Input: part model. Units: mm. Frame: model coordinates. Face numbers are marked on the shaded views. A direction names the side the tool comes from. Give positions to 0.01 mm unless a question says otherwise; leave off trailing zeros. Write each loop counter-clockwise with the first axis right and the second up, starting at its lowest first coordinate (ties: lowest second). Pieces come first, ordered by that corner, then holes. Notation, with made-up numbers: (77.5, -34.5) -> (97.5, -34.5) arc R13 ccw to (97.5, -19.5) -> close; hole circle Ø4 at (2, 25.5). An arc over 180 degrees is marked (long way). Answer as a JSON object with one key per item and string values. Group by question number.
from build123d import *

# Parameters (mm, degrees)
BOSS_EXTRUDE1_DEPTH = 5
SKETCH2_R           = 1.5
CUT_EXTRUDE1_DEPTH  = 5
SKETCH1_4_OUTSIDE_W = 53.856
SKETCH1_4_OUTSIDE_H = 58.288
SKETCH1_4_OUTSIDE_R = 1.5
CUT_EXTRUDE3_DEPTH  = 31.230173018
BOSS_EXTRUDE2_DEPTH = 40
SKETCH5_W           = 5
SKETCH5_H           = 50
BOSS_EXTRUDE3_DEPTH = 40
BOSS_EXTRUDE4_DEPTH = 40
SKETCH9_R           = 2
CUT_EXTRUDE4_DEPTH  = 84.384553352


with BuildPart() as part:
    # Sketch1 → Boss-Extrude1 (new body)
    with BuildSketch(Plane(origin=(0, 0, 0), x_dir=(1, 0, 0), z_dir=(0, 1, 0))):
        Polygon((-14.94438846, 22.160431622), (14.94438846, 22.160431622), (19.94438846, 17.160431622), (19.94438846, -22.160431622), (-19.94438846, -22.160431622), (-19.94438846, 17.160431622), align=None)
    extrude(amount=BOSS_EXTRUDE1_DEPTH)

    # Sketch2 → Cut-Extrude1 (cut)
    with BuildSketch(Plane.XZ):
        with Locations(Location((-8.780710157, 0, 0), (0, 0, 270))):
            Circle(SKETCH2_R)
    extrude(amount=-CUT_EXTRUDE1_DEPTH, mode=Mode.SUBTRACT)

    # Sketch1_4 outside → Cut-Extrude3 (cut, through all)
    # profile 1 of 3: a face of its own
    with BuildSketch(Plane(origin=(0, 0, 0), x_dir=(1, 0, 0), z_dir=(0, 1, 0))):
        Rectangle(SKETCH1_4_OUTSIDE_W, SKETCH1_4_OUTSIDE_H)
        Polygon((-14.94438846, 22.160431622), (14.94438846, 22.160431622), (19.94438846, 17.160431622), (19.94438846, -22.160431622), (-19.94438846, -22.160431622), (-19.94438846, 17.160431622), align=None, mode=Mode.SUBTRACT)
    # profile 2 of 3: a face of its own
    with BuildSketch(Plane(origin=(0, 0, 0), x_dir=(1, 0, 0), z_dir=(0, 1, 0))):
        with Locations(Location((8.788189679, 0, 0), (0, 0, 270))):
            Circle(SKETCH1_4_OUTSIDE_R)
    # profile 3 of 3: a face of its own
    with BuildSketch(Plane(origin=(0, 0, 0), x_dir=(1, 0, 0), z_dir=(0, 1, 0))):
        with Locations((-8.788189679, 0)):
            Circle(SKETCH1_4_OUTSIDE_R)
    extrude(amount=CUT_EXTRUDE3_DEPTH, mode=Mode.SUBTRACT)

    # Sketch4 → Boss-Extrude2 (add)
    with BuildSketch(Plane(origin=(19.94438846, 0, 0), x_dir=(0, 0, -1), z_dir=(1, 0, 0))):
        with BuildLine():
            Line((-22.160431622, 5), (-22.160431622, 0))
            ThreePointArc((-22.160431622, 0), (-29.231499434, 2.928932188), (-32.160431622, 10))
            Line((-32.160431622, 10), (-27.160431622, 10))
            ThreePointArc((-27.160431622, 10), (-25.695965528, 6.464466094), (-22.160431622, 5))
        make_face()
    extrude(amount=-BOSS_EXTRUDE2_DEPTH)

    # Sketch5 → Boss-Extrude3 (add)
    with BuildSketch(Plane(origin=(19.94438846, 0, 0), x_dir=(0, 0, -1), z_dir=(1, 0, 0))):
        with Locations((-29.660431622, 35)):
            Rectangle(SKETCH5_W, SKETCH5_H)
    extrude(amount=-BOSS_EXTRUDE3_DEPTH)

    # Sketch6 → Boss-Extrude4 (add)
    with BuildSketch(Plane(origin=(19.94438846, 0, 0), x_dir=(0, 0, -1), z_dir=(1, 0, 0))):
        Polygon((-10.08936381, 5), (-18.624897716, 13.535533906), (-27.160431622, 22.071067812), (-27.160431622, 17.071067812), (-15.08936381, 5), align=None)
    extrude(amount=-BOSS_EXTRUDE4_DEPTH)

    # Sketch9 → Cut-Extrude4 (cut, through all)
    with BuildSketch(Plane.XY.offset(32.160431622)):
        with Locations((-0.05561154, 46)):
            Circle(SKETCH9_R)
    extrude(amount=-CUT_EXTRUDE4_DEPTH, mode=Mode.SUBTRACT)


solid = part.part
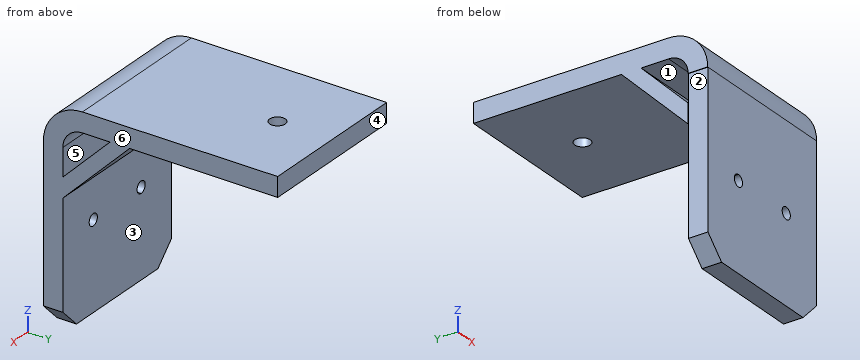
1. Reachability of the marked faces 1, 2 and 3 from +Z, -Z, +X, -X, +Y, -Y: full face, straight path, thin tool, end or side. Return the list, or none.
2. Contact query for flat-ended pins moving along their axis: pin 1 Ø1.5 at (y, z) = (2.5, -6.5) entering from -X; pin 2 Ø11.5 at (x, y) = (6.5, 44.5) entering from -Z; pin 3 Ø10 at (x, y) = (9, 23.5) entering from -Z; pin 4 Ø1.8 at (x, z) = (8.79, 0) entering from -Y. Output: stop coordinate, or through.
3. Section B-B (z = 0). Return the cut outline in (x, y).
4. Mould query, pull axis Y, two halves, no side actions, for the marked faces 4, 5 and 6. Classes: pulls with the +Y half, pulls with the -Y half, needs draft (parallel to the pull), parting line crosses it, or undercut.
5. Section C-C (y = 46). Return the cut outline in (x, z), plus the area to 3 significant figures.
6. Line query: line 1 (X direction, y = 1, z = 0); line 2 (Z direction, x = -14, y = 52); line 3 (Y direction, x = -17, z = -7). Output: solid intervals per line, ascending.
7. Section D-D (x = 0). Return the cut outline in (y, z), plus the area to 3 significant figures.
8. Section A-A (x = 14). Return the cut outline in (y, z).
Working result:
{
 "1": {"face 1": "+X, -X", "face 2": "-Z, -X, -Y", "face 3": "-Z, +X, -X, +Y"},
 "2": {"pin 1": "stops at x = -19.94", "pin 2": "stops at z = 27.16", "pin 3": "stops at z = 23.59", "pin 4": "passes through"},
 "3": {"outline": "(-19.94, 0) -> (-10.29, 0) -> (-10.29, 5) -> (-19.94, 5) -> close; (-7.28, 0) -> (7.29, 0) -> (7.29, 5) -> (-7.28, 5) -> close; (10.29, 0) -> (19.94, 0) -> (19.94, 5) -> (10.29, 5) -> close"},
 "4": {"face 4": "pulls with the +Y half", "face 5": "undercut", "face 6": "needs draft"},
 "5": {"outline": "(-20.06, 27.16) -> (-2.06, 27.16) -> (-2.06, 32.16) -> (-20.06, 32.16) -> close; (1.94, 27.16) -> (19.94, 27.16) -> (19.94, 32.16) -> (1.94, 32.16) -> close", "area": "180 mm^2"},
 "6": {"line 1": "x = -19.94 to -10.29, -7.28 to 7.29, 10.29 to 19.94", "line 2": "z = 27.16 to 32.16", "line 3": "y = 0 to 5"},
 "7": {"outline": "(0, -22.16) -> (5, -22.16) -> (5, 10.09) -> (22.07, 27.16) -> (44, 27.16) -> (44, 32.16) -> (10, 32.16) arc R10 ccw to (0, 22.16) -> close; (48, 27.16) -> (60, 27.16) -> (60, 32.16) -> (48, 32.16) -> close; hole (5, 15.09) -> (17.07, 27.16) -> (10, 27.16) arc R5 ccw to (5, 22.16) -> close", "area": "583 mm^2"},
 "8": {"outline": "(0, -22.16) -> (5, -22.16) -> (5, 10.09) -> (22.07, 27.16) -> (60, 27.16) -> (60, 32.16) -> (10, 32.16) arc R10 ccw to (0, 22.16) -> close; hole (5, 15.09) -> (17.07, 27.16) -> (10, 27.16) arc R5 ccw to (5, 22.16) -> close"}
}
